Can you work these out from the model? Positions are in its coordinate system, mm. Face numbers are marked on the shaded views. Give positions to 0.01 mm unless a question says otherwise; leave off trailing zeros. Order: outer loops, then holes, each group sorted by start corner. A loop starts at its lowest first (then second) coordinate and runs counter-clockwise, first axis right, second up. Notation, with made-up numbers: (65.5, 50.25) - (85.5, 50.25) arc R18 ccw to (85.5, 66.25) - close; hole circle Ø7 at (-10.5, -32). An arc over 180 degrees is marked (long way). One line per question, with ' | ' between items.
```python
from build123d import *

# Parameters (mm, degrees)
F2_DEPTH = 5


with BuildPart() as f2:
    # F1 (on Right) → F2 (new body)
    with BuildSketch(Plane.YZ):
        Polygon((0, 5), (0, 0), (31.5, 0), (31.5, -5), (36.5, -5), (36.5, 0), (45, 0), (45, 2), (43.75, 2), (43.75, 5), (45, 5), (45, 6), (48, 6), (48, 5), (49.25, 5), (49.25, 2), (48, 2), (48, 0), (56.5, 0), (56.5, -5), (61.5, -5), (61.5000005474, 0), (93, 0), (93, 5), (98, 5), (98, 10), (93, 10), (93, 18.5), (91, 18.5), (91, 17.25), (88, 17.25), (88, 18.5), (87, 18.5), (87, 21.5), (88, 21.5), (88, 22.75), (91, 22.75), (91, 21.5), (93, 21.5), (93, 30), (98, 30), (98, 35), (93, 35), (93, 40), (61.5000005474, 40), (61.5, 45), (56.5, 45), (56.5, 40), (48, 40), (48, 38), (49.25, 38), (49.25, 35), (48, 35), (48, 34), (45, 34), (45, 35), (43.75, 35), (43.75, 38), (45, 38), (45, 40), (36.5, 40), (36.5, 45), (31.5, 45), (31.5, 40), (0, 40), (0, 35), (-5, 35), (-5, 30), (0, 30), (0, 21.5), (2, 21.5), (2, 22.75), (5, 22.75), (5, 21.5), (6, 21.5), (6, 18.5), (5, 18.5), (5, 17.25), (2, 17.25), (2, 18.5), (0, 18.5), (0, 10), (-5, 10), (-5, 5), align=None)
    extrude(amount=F2_DEPTH)


solid = f2.part
```
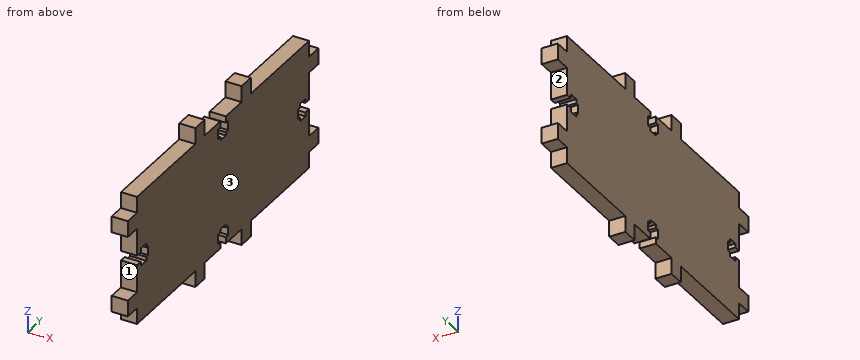
(1) Imagine slicing it at B-B (z = 42). List the corners of the cut face in (x, y) for me, and give its area (3 significant figures).
Answer below:
outline: (0, 31.5) - (5, 31.5) - (5, 36.5) - (0, 36.5) - close; (0, 56.5) - (5, 56.5) - (5, 61.5) - (0, 61.5) - close | area: 50.0 mm^2
(2) Will these pins go through, and if not, where does the flat tip stop? pin 1 (1.5 mm diameter, centred on x = 3, y = 96.5, fed in from +Z); pin 2 (0.6 mm diameter, centred on x = 1.5, y = 48.5, fed in from +Z); pin 3 (2 mm diameter, centred on x = 1.5, z = 39, fed in from +Y).
Answer below:
pin 1: z = 35 | pin 2: z = 40 | pin 3: y = 93
(3) Imagine slicing it at D-D (y = 16.5). List the corners of the cut face in (x, z) for me, and give its area (3 significant figures).
Answer below:
outline: (0, 0) - (5, 0) - (5, 40) - (0, 40) - close | area: 200 mm^2
(4) If we mould it in two halves opening along Z, with no side actions, what happens to the marked faces 1, 2 and 3? For each: released by +Z, released by -Z, zero draft, split by the parting line, or undercut.
Answer below:
face 1: undercut | face 2: undercut | face 3: zero draft
(5) If I drill on line 1 (Z direction, x = 3.9, y = 44); line 2 (Z direction, x = 3.2, y = 92.5); line 3 (Y direction, x = 4.5, z = 1), over which ranges is the centre line in solid material (lowest first)?
Answer below:
line 1: 0 to 2, 5 to 35, 38 to 40 | line 2: 0 to 18.5, 21.5 to 40 | line 3: 0 to 45, 48 to 93
(6) Imagine slicing it at A-A (y = 90). List the corners of the cut face in (x, z) for me, and give its area (4 significant figures).
Answer below:
outline: (0, 0) - (5, 0) - (5, 17.25) - (0, 17.25) - close; (0, 22.75) - (5, 22.75) - (5, 40) - (0, 40) - close | area: 172.5 mm^2
(7) Imagine slicing it at C-C (z = 26). List the corners of the cut face in (x, y) for me, and give its area (3 significant figures).
Answer below:
outline: (0, 0) - (5, 0) - (5, 93) - (0, 93) - close | area: 465 mm^2
